Design review of the part built by this model. Coordinates are the model's own, in mm. A direction names the side the tool comes from. Give positions to 0.01 mm unless a question says otherwise; leave off trailing zeros. Loops run counter-clockwise (first coordinate to the right, second up) from the corner with the lowest first, then second, coordinate; pieces in that order, holes last. Notation, with made-up numbers: M 42,-6.75 L 72,-6.75 A21 ccw 72,19.25 Z; hole C 2.5,36 d5. An arc over 180 degrees is marked long. Use a Markdown table: item, result. Add a question column.
(1) For probe 1 along Z at (x, y) = (24.5, 89); probe 2 along X at (y, z) = (12, 4); probe 3 along Y at (x, z) = (-15.5, 13.5), list the stretches that pass through material, from the lowest coordinate up.
(2) Add section B-B, the plane y = 29.5. Give the boundary of the cut face in (x, z).
(3) Add section A-A, the plane x = -15. Give the boundary of the cut face in (y, z).
(4) For faces 1 (the face through (-14, 14, 8)), 2 (the face through (-18, -2, 8.8)), 3 (the face through (-10, 7, 8)), 4 (the face through (-18, 7, 8)), list the 3-axis set-ups (+Z, -Z, +X, -X, +Y, -Y) from which the entire face can be reached by the end or side of a thin tool; tool diameter is ignored.
(5) Add section C-C, the plane x = 21. Give the boundary of the cut face in (y, z), then the cut area to 3 significant figures.
(6) Insertion check: pin 1 Ø4 at (y, z) = (46.5, 3) entering from -X; pin 2 Ø4.5 at (x, z) = (-11, 4) entering from -Y; pin 3 Ø4 at (y, z) = (5.5, 8) entering from -X. Each pin has a flat end and moves straight along its axis. Give the tip position at first contact, or say it passes through.
```python
from build123d import *

# Parameters (mm, degrees)
F0_W     = 66
F0_H     = 97
F1_DEPTH = 1.6
F2_W     = 8
F2_H     = 14
F3_DEPTH = 12.6
F5_DEPTH = 4


with BuildPart() as f1:
    # F0 (on Top) → F1 (new body)
    with BuildSketch(Plane.XY):
        with Locations((0, 48.5)):
            Rectangle(F0_W, F0_H)
    extrude(amount=F1_DEPTH)

    # F2 (on face) → F3 (join)
    with BuildSketch(Plane.XY.offset(1.6)):
        with Locations((-14, 7)):
            Rectangle(F2_W, F2_H)
    extrude(amount=F3_DEPTH)

    # F4 (on face) → F5 (join)
    with BuildSketch(Plane.XZ):
        with BuildLine():
            ThreePointArc((-18, 8.7), (-15, 5.7), (-12, 8.7))
            ThreePointArc((-12, 8.7), (-15, 11.7), (-18, 8.7))
        make_face()
    extrude(amount=F5_DEPTH)


solid = f1.part
```
Established:
| question | item | result |
|---|---|---|
| 1 | probe 1 | 0 to 1.6 |
| 1 | probe 2 | -18 to -10 |
| 1 | probe 3 | 0 to 14 |
| 2 | outline | M -33,0 L 33,0 L 33,1.6 L -33,1.6 Z |
| 3 | outline | M -4,5.7 L 0,5.7 L 0,0 L 97,0 L 97,1.6 L 14,1.6 L 14,14.2 L 0,14.2 L 0,11.7 L -4,11.7 Z |
| 4 | face 1 | +Z, +X, -X, +Y |
| 4 | face 2 | -Y |
| 4 | face 3 | +Z, +X, +Y, -Y |
| 4 | face 4 | +Z, -X, +Y, -Y |
| 5 | outline | M 0,0 L 97,0 L 97,1.6 L 0,1.6 Z |
| 5 | area | 155 mm^2 |
| 6 | pin 1 | x = -33 |
| 6 | pin 2 | y = 0 |
| 6 | pin 3 | x = -18 |
